Could you check a few things on this drawing? It's one solid part, dimensions in mm from its lowest x, y, z. A direction names the side the tool comes from. Coordinates: 2 decimals unless noted, no trailing zeros. Order: outer loops, then holes, each group sorted by start corner. A loop starts at its lowest first (then second) coordinate and runs counter-clockwise, first axis right, second up. Notation, with made-up numbers: M 47.25,84 L 92.25,84 A32 ccw 92.25,112 Z; hole C 38,-8.75 d11. An arc over 180 degrees is marked long. Answer as CSV lines item,"result". Start each with the question number.
1. If we section it at C-C (z = 1.5): List the corners of the cut face in (x, y) for me, plus the area to 4 significant figures.
2. Will these pins go through, and if not, where does the flat tip stop? pin 1 (2.5 mm diameter, centred on x = 9, z = 9, fed in from +Y); pin 2 (2.5 mm diameter, centred on y = 25, z = 5, fed in from +X); pin 3 (1.5 mm diameter, centred on y = 12.5, z = 2, fed in from -X); pin 4 (10 mm diameter, centred on x = 7.5, y = 16.5, fed in from +Z).
3. On a 3-axis mill with a long thin cutter (end or side, diameter ignored), from which of +Z, -Z, +X, -X, +Y, -Y can I reach the whole of each face in a straight line? I mean the marked faces 5, 6 and 7. Say none if no direction works.
4. If we section it at A-A (y = 25): List the corners of the cut face in (x, z) for me.
5. If we section it at D-D (y = 21.5): List the corners of the cut face in (x, z) for me, plus the area to 3 significant figures.
6. If we mould it in two halves opening along X, with no side actions, what happens to the marked faces 1, 2, 3 and 4? For each: released by +X, released by -X, zero draft, split by the parting line, or undercut.
7. I need wall thicknesses on line 1 along X through (y, z) = (28.7, 9); line 2 along Z through (x, y) = (0.45, 25); line 3 along Z through (x, y) = (23.1, 1.5). Which ranges of each line are inside material? Lowest first, please. Write a range as from..to.
8. If we section it at B-B (x = 9): List the corners of the cut face in (y, z) for me, plus the area to 3 significant figures.
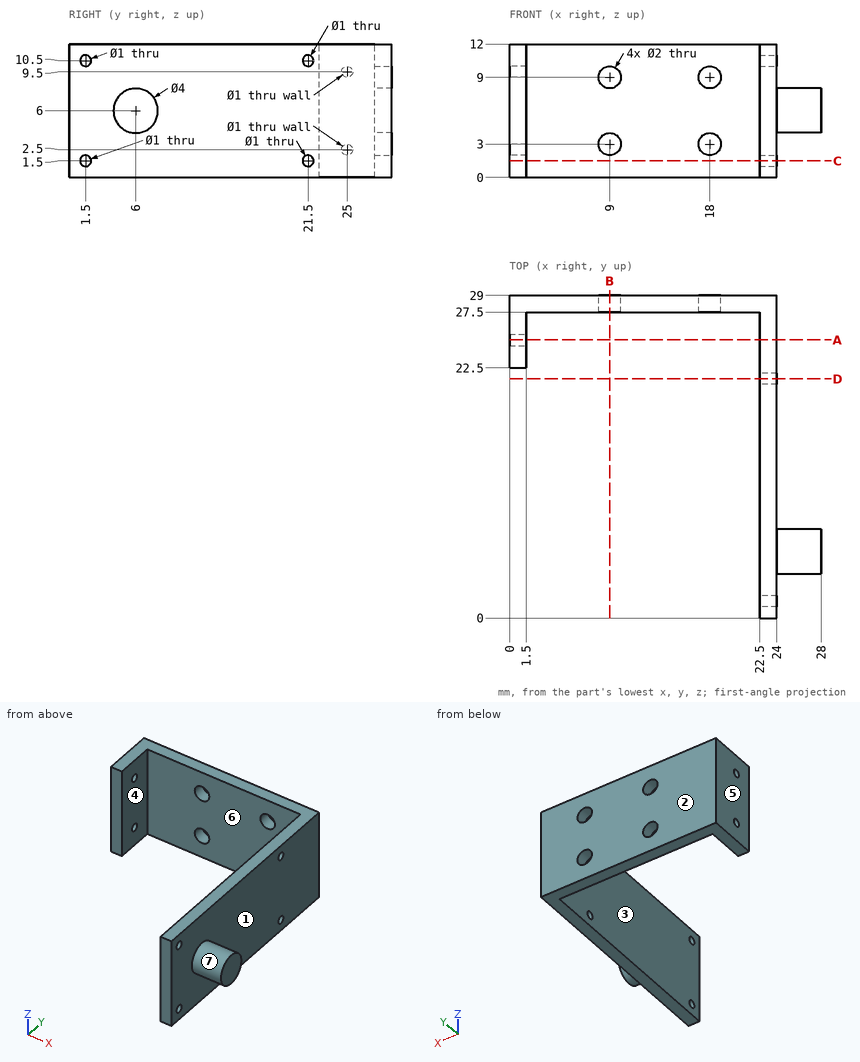
Solved:
1,outline,"M 0,22.5 L 1.5,22.5 L 1.5,27.5 L 22.5,27.5 L 22.5,22 L 24,22 L 24,29 L 0,29 Z; M 22.5,0 L 24,0 L 24,1 L 22.5,1 Z; M 22.5,2 L 24,2 L 24,21 L 22.5,21 Z"
1,area,"81.75 mm²"
2,pin 1,"y = 29"
2,pin 2,"x = 24"
2,pin 3,"x = 22.5"
2,pin 4,"through"
3,face 5,"+Z, -Z, -X, +Y, -Y"
3,face 6,"+Z, -Z, -Y"
3,face 7,"+X"
4,outline,"M 0,0 L 1.5,0 L 1.5,2 L 0,2 Z; M 0,3 L 1.5,3 L 1.5,9 L 0,9 Z; M 0,10 L 1.5,10 L 1.5,12 L 0,12 Z; M 22.5,0 L 24,0 L 24,12 L 22.5,12 Z"
5,outline,"M 22.5,0 L 24,0 L 24,1 L 22.5,1 Z; M 22.5,2 L 24,2 L 24,10 L 22.5,10 Z; M 22.5,11 L 24,11 L 24,12 L 22.5,12 Z"
5,area,"15.0 mm²"
6,face 1,"released by +X"
6,face 2,"zero draft"
6,face 3,"undercut"
6,face 4,"undercut"
7,line 1,"0..8, 10..17, 19..24"
7,line 2,"0..2, 3..9, 10..12"
7,line 3,"0..1, 2..10, 11..12"
8,outline,"M 27.5,0 L 29,0 L 29,2 L 27.5,2 Z; M 27.5,4 L 29,4 L 29,8 L 27.5,8 Z; M 27.5,10 L 29,10 L 29,12 L 27.5,12 Z"
8,area,"12.0 mm²"
